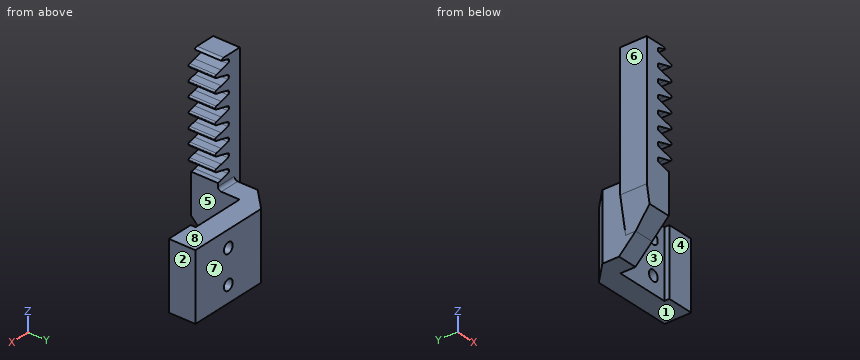
from build123d import *

# Parameters (mm, degrees)
SKETCH1_W           = 30
SKETCH1_H           = 16
BOSS_EXTRUDE1_DEPTH = 20
CUT_EXTRUDE1_DEPTH  = 20
SKETCH3_W           = 6
SKETCH3_H           = 10
BOSS_EXTRUDE2_DEPTH = 5
SKETCH9_R           = 1.6
CUT_EXTRUDE3_DEPTH  = 6.5
SKETCH11_W          = 10
SKETCH11_H          = 8
BOSS_EXTRUDE4_DEPTH = 40
CHAMFER2_SIZE2      = 10
CHAMFER2_SIZE       = 2
FILLET1_R           = 1
CUT_EXTRUDE4_DEPTH  = 8
SKETCH13_W          = 2
SKETCH13_H          = 8
BOSS_EXTRUDE5_DEPTH = 10
LPATTERN1_COUNT     = 8
LPATTERN1_PITCH     = 4.25
FILLET2_R           = 0.5
FILLET3_R           = 1
SKETCH14_W          = 2
SKETCH14_H          = 8
CUT_EXTRUDE5_DEPTH  = 17
CHAMFER3_SIZE       = 6
CHAMFER4_SIZE       = 5


# Some blends are built 0.0001 mm under size
with BuildPart() as part:
    # Sketch1 → Boss-Extrude1 (new body)
    with BuildSketch(Plane.XY):
        with Locations((15, -8)):
            Rectangle(SKETCH1_W, SKETCH1_H)
    extrude(amount=BOSS_EXTRUDE1_DEPTH)

    # Sketch2 → Cut-Extrude1 (cut)
    with BuildSketch(Plane.XY.offset(20)):
        Polygon((22, -6.5), (22, -8), (30, -8), (30, -16), (6, -16), (6, -6.5), align=None)
    extrude(amount=-CUT_EXTRUDE1_DEPTH, mode=Mode.SUBTRACT)

    # Sketch3 → Boss-Extrude2 (add)
    with BuildSketch(Plane.XZ.offset(16)):
        with Locations((3, 10)):
            Rectangle(SKETCH3_W, SKETCH3_H)
    extrude(amount=BOSS_EXTRUDE2_DEPTH)

    # Sketch9 → Cut-Extrude3 (cut)
    with BuildSketch(Plane.XZ.offset(6.5)):
        with Locations(Location((18, 15, 0), (0, 0, 270))):
            Circle(SKETCH9_R)
        with Locations(Location((18, 5, 0), (0, 0, 270))):
            Circle(SKETCH9_R)
    extrude(amount=-CUT_EXTRUDE3_DEPTH, mode=Mode.SUBTRACT)

    # Sketch11 → Boss-Extrude4 (add)
    with BuildSketch(Plane.XY.offset(15)):
        with Locations((3, -17)):
            Rectangle(SKETCH11_W, SKETCH11_H)
    extrude(amount=BOSS_EXTRUDE4_DEPTH)

    # Chamfer2
    chamfer2_edges = [part.edges().sort_by_distance(p)[0] for p in [
        (0, -17, 15),
    ]]
    chamfer2_side = [part.faces().sort_by_distance(p)[0] for p in [
        (-0.04, -17, 15),
    ]]
    chamfer(chamfer2_edges, length=CHAMFER2_SIZE - 0.0001, length2=CHAMFER2_SIZE2 - 0.0001, reference=chamfer2_side[0])  # a hair under: the kernel refuses the full size

    # Fillet1
    fillet1_edges = [part.edges().sort_by_distance(p)[0] for p in [
        (3, -13, 20),
    ]]
    fillet(fillet1_edges, radius=FILLET1_R)

    # Sketch12 → Cut-Extrude4 (cut)
    with BuildSketch(Plane.XZ.offset(21)):
        Polygon((7, 55), (4.75, 54.5), (2, 53.75), (2, 52.75), (4.75, 52), (7, 51.5), (7, 50.75), (8, 50.75), (8, 55), align=None)
    cut_extrude4 = extrude(amount=-CUT_EXTRUDE4_DEPTH, mode=Mode.SUBTRACT)

    # Sketch13 → Boss-Extrude5 (add)
    with BuildSketch(Plane(origin=(0, 0, 15), x_dir=(-1, 0, 0), z_dir=(0, 0, -1))):
        with Locations((-7, -17)):
            Rectangle(SKETCH13_W, SKETCH13_H)
    extrude(amount=BOSS_EXTRUDE5_DEPTH)

    # LPattern1: Cut-Extrude4 ×8
    with Locations(*[(0, 0, -i * LPATTERN1_PITCH) for i in range(1, LPATTERN1_COUNT)]):
        add(cut_extrude4, mode=Mode.SUBTRACT)

    # Fillet2
    # the kernel refuses this fillet: 0.5 mm, written as the material it adds along each edge
    with BuildSketch(Plane(origin=(2, -21, 52.75), x_dir=(0.9647638212377322, 0, -0.26311740579210835), z_dir=(0, 1, 0)), Plane(origin=(2, -21, 53.75), x_dir=(0, 0, -1), z_dir=(0, 1, 0)), Plane(origin=(2, -21, 48.5), x_dir=(0.9647638212377321, 0, -0.26311740579210924), z_dir=(0, 1, 0)), Plane(origin=(2, -21, 49.5), x_dir=(0, 0, -1), z_dir=(0, 1, 0)), Plane(origin=(2, -21, 44.25), x_dir=(0.9647638212377321, 0, -0.26311740579210924), z_dir=(0, 1, 0)), Plane(origin=(2, -21, 45.25), x_dir=(0, 0, -1), z_dir=(0, 1, 0)), Plane(origin=(2, -21, 35.75), x_dir=(0.9647638212377321, 0, -0.26311740579210896), z_dir=(0, 1, 0)), Plane(origin=(2, -21, 36.75), x_dir=(0, 0, -1), z_dir=(0, 1, 0)), Plane(origin=(2, -21, 40), x_dir=(0.9647638212377321, 0, -0.26311740579210924), z_dir=(0, 1, 0)), Plane(origin=(2, -21, 41), x_dir=(0, 0, -1), z_dir=(0, 1, 0)), Plane(origin=(2, -21, 23), x_dir=(0.9647638212377319, 0, -0.2631174057921095), z_dir=(0, 1, 0)), Plane(origin=(2, -21, 24), x_dir=(0, 0, -1), z_dir=(0, 1, 0)), Plane(origin=(2, -21, 27.25), x_dir=(0.9647638212377319, 0, -0.2631174057921095), z_dir=(0, 1, 0)), Plane(origin=(2, -21, 28.25), x_dir=(0, 0, -1), z_dir=(0, 1, 0)), Plane(origin=(2, -21, 32.5), x_dir=(0, 0, -1), z_dir=(0, 1, 0)), Plane(origin=(2, -21, 31.5), x_dir=(0.9647638212377319, 0, -0.2631174057921095), z_dir=(0, 1, 0))) as fillet2_piece_1:
        with BuildLine():
            CenterArc((FILLET2_R * 0.763795840999, -FILLET2_R), FILLET2_R, 90, 74.744881297)
            Line((-FILLET2_R * 0.200967980239, -FILLET2_R * 0.736882594208), (0, 0))
            Line((0, 0), (FILLET2_R * 0.763795840999, 0))
        make_face()
    extrude(amount=8)
    # the kernel refuses this fillet: 0.5 mm, written as the material it takes off along each edge
    with BuildSketch(Plane(origin=(7, -22.002714508, 33.75), x_dir=(-0.9761870601839541, 0, -0.21693045781865056), z_dir=(0, 1, 0)), Plane(origin=(7, -22.002714508, 34.5), x_dir=(0, 0, -1), z_dir=(0, 1, 0)), Plane(origin=(7, -22.002714508, 38), x_dir=(-0.9761870601839535, 0, -0.21693045781865242), z_dir=(0, 1, 0)), Plane(origin=(7, -22.002714508, 38.75), x_dir=(0, 0, -1), z_dir=(0, 1, 0)), Plane(origin=(7, -22.002714508, 42.25), x_dir=(-0.9761870601839538, 0, -0.216930457818651), z_dir=(0, 1, 0)), Plane(origin=(7, -22.002714508, 43), x_dir=(0, 0, -1), z_dir=(0, 1, 0)), Plane(origin=(7, -22.002714508, 46.5), x_dir=(-0.9761870601839538, 0, -0.216930457818651), z_dir=(0, 1, 0)), Plane(origin=(7, -22.002714508, 47.25), x_dir=(0, 0, -1), z_dir=(0, 1, 0)), Plane(origin=(7, -22.002714508, 50.75), x_dir=(-0.9761870601839538, 0, -0.216930457818651), z_dir=(0, 1, 0)), Plane(origin=(7, -22.002714508, 51.5), x_dir=(0, 0, -1), z_dir=(0, 1, 0)), Plane(origin=(7, -22.002714508, 25.25), x_dir=(-0.9761870601839521, 0, -0.21693045781865947), z_dir=(0, 1, 0)), Plane(origin=(7, -22.002714508, 26), x_dir=(0, 0, -1), z_dir=(0, 1, 0)), Plane(origin=(7, -22.002714508, 29.5), x_dir=(-0.9761870601839522, 0, -0.2169304578186585), z_dir=(0, 1, 0)), Plane(origin=(7, -22.002714508, 30.25), x_dir=(0, 0, -1), z_dir=(0, 1, 0))) as fillet2_2_piece_1:
        with BuildLine():
            CenterArc((FILLET2_R * 0.802171606366, FILLET2_R), FILLET2_R, 192.528807709, 77.471192291)
            Line((-FILLET2_R * 0.174015453818, FILLET2_R * 0.783069542181), (0, 0))
            Line((0, 0), (FILLET2_R * 0.802171606366, 0))
        make_face()
    extrude(amount=10.005429016, mode=Mode.SUBTRACT)

    # Fillet3
    # the kernel refuses this fillet: 1 mm, written as the material it takes off along each edge
    with BuildSketch(Plane(origin=(7, -28.790063509, 55), x_dir=(-1, 0, 0), z_dir=(0, 1, 0))) as fillet3_piece_1:
        with BuildLine():
            CenterArc((3.116025404, -1), FILLET3_R, 90, 60)
            Line((2.25, -0.5), (0, 0))
            Line((0, 0), (3.116025404, 0))
        make_face()
    extrude(amount=23.580127019, mode=Mode.SUBTRACT)

    # Sketch14 → Cut-Extrude5 (cut)
    with BuildSketch(Plane(origin=(0, 0, 5), x_dir=(-1, 0, 0), z_dir=(0, 0, -1))):
        with Locations((-7, -17)):
            Rectangle(SKETCH14_W, SKETCH14_H)
    extrude(amount=-CUT_EXTRUDE5_DEPTH, mode=Mode.SUBTRACT)

    # Chamfer3
    chamfer3_edges = [part.edges().sort_by_distance(p)[0] for p in [
        (0, 0, 10),
    ]]
    chamfer(chamfer3_edges, length=CHAMFER3_SIZE)

    # Chamfer4
    chamfer4_edges = [part.edges().sort_by_distance(p)[0] for p in [
        (3, -21, 5),
        (3, -16, 0),
    ]]
    chamfer(chamfer4_edges, length=CHAMFER4_SIZE - 0.0001)  # a hair under: the kernel refuses the full size


solid = part.part
Part model, mm, in its own coordinate system. Face numbers are marked on the shaded views. A direction names the side the tool comes from. Give positions to 0.01 mm unless a question says otherwise; leave off trailing zeros. Order: outer loops, then holes, each group sorted by start corner. A loop starts at its lowest first (then second) coordinate and runs counter-clockwise, first axis right, second up. Notation, with made-up numbers: (87, -30) -> (111, -30) arc R28 ccw to (111, -3) -> close; hole circle Ø4 at (-23.75, 80.25). An arc over 180 degrees is marked (long way). Use one line per item in the form item = value.
(1) Flat gauge pins, fed straight in: P1, Ø1.9, axis at x = 18, z = 15, coming from the -Y side; P2, Ø6, axis at x = 20, y = -6, coming from the +Z side; P3, Ø10, axis at x = 2, y = -18, coming from the -Z side; P4, Ø8, axis at y = -13, z = 5.5, coming from the -X side. Where does each tip first touch, or does it go through?
Solution:
P1 = through
P2 = 20
P3 = 2
P4 = -0.9
(2) Tool access for the marked faces 4, 5, 6, 7 and 8: list every direction of +Z, -Z, +X, -X, +Y, -Y with a clear straight run to the whole face (end or side of a thin tool).
Solution:
face_4 = +Z, -Z, +X, -Y
face_5 = -Z, -Y
face_6 = +Z, -Z, -X, +Y, -Y
face_7 = +Z, -Z, +X, -X, +Y
face_8 = +Z, +X, -X, +Y
(3) Drill centre lines: line 1 (Y direction, x = 20, z = 15); line 2 (X direction, y = -3.75, z = 15); line 3 (Z direction, x = 26, y = -5.5). Where is each one in solid material? Low to high. Write a range as from..to.
Solution:
line_1 = -6.5..0
line_2 = 2.25..16.4, 19.6..30
line_3 = 0..20
(4) Saw through at A-A (y = -3.75). Write the cut outline in (x, z), then the cut area to 3 significant figures.
Solution:
outline = (2.25, 0) -> (30, 0) -> (30, 20) -> (2.25, 20) -> close; hole circle Ø3.2 at (18, 5); hole circle Ø3.2 at (18, 15)
area = 539 mm²
(5) Pull direction X, two halves, no side cores. Call the marked faces 1, 2 and 3: +X half, -X half, draft (parallel to the pull), parting line (faces both ways), or undercut.
Solution:
face_1 = draft
face_2 = +X half
face_3 = undercut
(6) Saw through at B-B (x = 18). Write the cut outline in (y, z).
Solution:
outline = (-6.5, 0) -> (0, 0) -> (0, 3.4) -> (-6.5, 3.4) -> close; (-6.5, 6.6) -> (0, 6.6) -> (0, 13.4) -> (-6.5, 13.4) -> close; (-6.5, 16.6) -> (0, 16.6) -> (0, 20) -> (-6.5, 20) -> close
(7) Saw through at C-C (x = 27.5). Write the cut outline in (y, z), then the cut area to 3 significant figures.
Solution:
outline = (-8, 0) -> (0, 0) -> (0, 20) -> (-8, 20) -> close
area = 160 mm²
